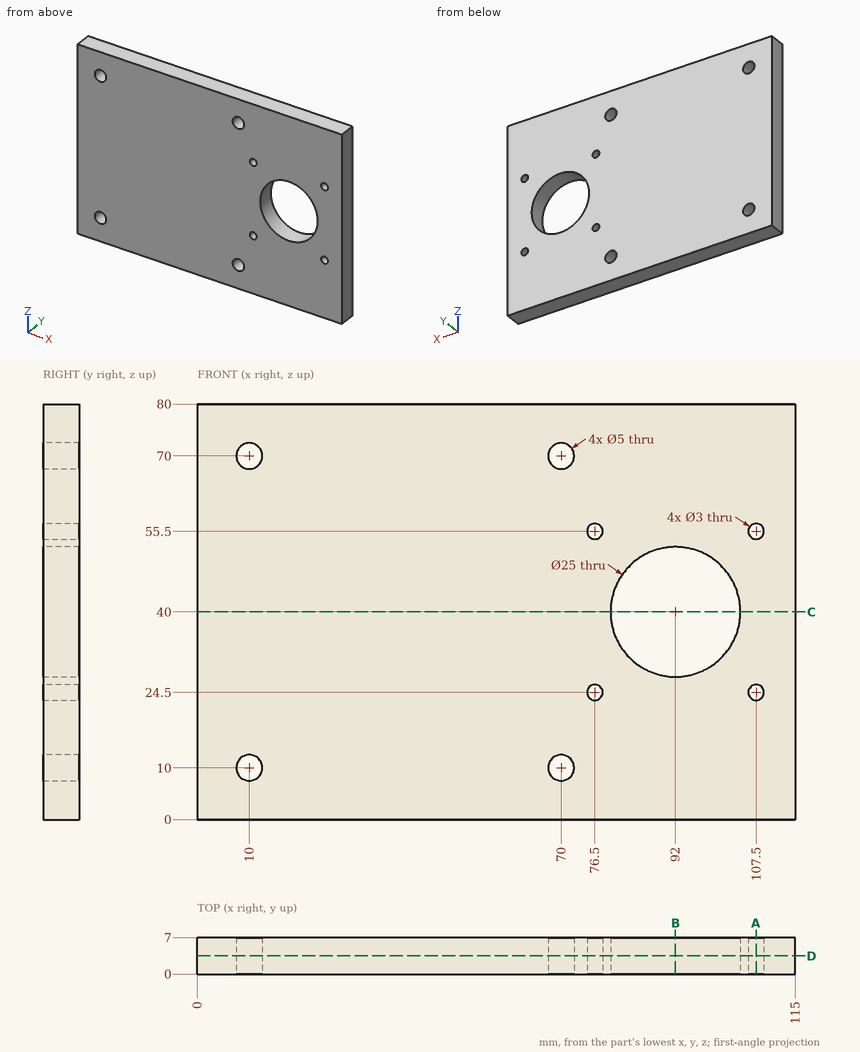
Answer from the drawing. Dimensions are ordinates in mm from the lowest x, y and z of the part. Give positions to 0.01 mm unless a question says otherwise; leave off trailing zeros. Order: outer loops, then holes, each group sorted by start corner. A loop starts at its lowest first (then second) coordinate and runs counter-clockwise, first axis right, second up.
(1) Find section D-D (y = 3.5). Give the number of separate pieces and of enclosed holes in the cut face, plus the area to 3 significant figures.
(2) Given pin 1 (4 mm diameter, centred on x = 70, z = 10, fed in from -Y), flat-ended and moving along its own axis, determine where the tip first touches the part or whether it passes through.
(3) Straight lines are drawn through the part: L1, parallel to Z at x = 76.5, y = 4.25; L2, parallel to X at y = 3.5, z = 55.5; L3, parallel to X at y = 5.5, z = 70. For each, find the intervals that lie inside material, in ascending order.
(4) Find section C-C (z = 40). Give the vertices of the cut face in (x, y).
(5) Find section B-B (x = 92). Give the vertices of the cut face in (y, z), plus the area to 3 significant figures.
(6) Find section A-A (x = 107.5). Give the vertices of the cut face in (y, z).
Result sheet:
1. separate pieces: 1
1. enclosed holes: 9
1. area: 8,600 mm2
2. pin 1: passes through
3. L1: z = 0 to 23, 26 to 54, 57 to 80
3. L2: x = 0 to 75, 78 to 106, 109 to 115
3. L3: x = 0 to 7.5, 12.5 to 67.5, 72.5 to 115
4. outline: (0, 0) - (79.5, 0) - (79.5, 7) - (0, 7) - close; (104.5, 0) - (115, 0) - (115, 7) - (104.5, 7) - close
5. outline: (0, 0) - (7, 0) - (7, 27.5) - (0, 27.5) - close; (0, 52.5) - (7, 52.5) - (7, 80) - (0, 80) - close
5. area: 385 mm2
6. outline: (0, 0) - (7, 0) - (7, 23) - (0, 23) - close; (0, 26) - (7, 26) - (7, 54) - (0, 54) - close; (0, 57) - (7, 57) - (7, 80) - (0, 80) - close
